from build123d import *

# Parameters (mm, degrees)
BOSS_EXTRUDE1_DEPTH = 2.54


with BuildPart() as part:
    # Sketch1 → Boss-Extrude1 (new body)
    with BuildSketch(Plane.XY):
        with BuildLine():
            Line((-109.2454, -66.7), (-109.2454, 67.7))
            ThreePointArc((-109.2454, 67.7), (-104.516521825, 79.116521825), (-93.1, 83.8454))
            Line((-93.1, 83.8454), (92.1, 83.8454))
            Line((92.1, 83.8454), (93.1, 83.8454))
            ThreePointArc((93.1, 83.8454), (104.516521825, 79.116521825), (109.2454, 67.7))
            Line((109.2454, 67.7), (109.2454, -66.7))
            Line((109.2454, -66.7), (109.2454, -67.7))
            ThreePointArc((109.2454, -67.7), (104.516521825, -79.116521825), (93.1, -83.8454))
            Line((93.1, -83.8454), (-92.1, -83.8454))
            Line((-92.1, -83.8454), (-93.1, -83.8454))
            ThreePointArc((-93.1, -83.8454), (-104.516521825, -79.116521825), (-109.2454, -67.7))
            Line((-109.2454, -67.7), (-109.2454, -66.7))
        make_face()
        with BuildLine():
            Line((-104.6734, -66.7), (-104.6734, 67.7))
            ThreePointArc((-104.6734, 67.7), (-101.283629621, 75.883629621), (-93.1, 79.2734))
            Line((-93.1, 79.2734), (92.1, 79.2734))
            Line((92.1, 79.2734), (93.1, 79.2734))
            ThreePointArc((93.1, 79.2734), (101.283629621, 75.883629621), (104.6734, 67.7))
            Line((104.6734, 67.7), (104.6734, -66.7))
            Line((104.6734, -66.7), (104.6734, -67.7))
            ThreePointArc((104.6734, -67.7), (101.283629621, -75.883629621), (93.1, -79.2734))
            Line((93.1, -79.2734), (-92.1, -79.2734))
            Line((-92.1, -79.2734), (-93.1, -79.2734))
            ThreePointArc((-93.1, -79.2734), (-101.283629621, -75.883629621), (-104.6734, -67.7))
            Line((-104.6734, -67.7), (-104.6734, -66.7))
        make_face(mode=Mode.SUBTRACT)
    extrude(amount=-BOSS_EXTRUDE1_DEPTH)


solid = part.part
Here's how the part is built. I have some questions about the finished solid (model axes, mm). A direction names the side the tool comes from. Round coordinates to 2 decimals unless told otherwise and drop trailing zeros. Order: outer loops, then holes, each group sorted by start corner. A loop starts at its lowest first (then second) coordinate and runs counter-clockwise, first axis right, second up. Notation, with made-up numbers: (55.5, 78.25) -> (61.5, 78.25) arc R30 cw to (61.5, 116.25) -> close; hole circle Ø5 at (67, 1). An arc over 180 degrees is marked (long way). Return JSON: item names as keys, results as strings.
Q1. If we section it at B-B on y = -7.5: List the corners of the cut face in (x, z) for me, plus the area to 3 significant figures.
Filled sheet:
{"outline": "(-109.25, -2.54) -> (-104.67, -2.54) -> (-104.67, 0) -> (-109.25, 0) -> close; (104.67, -2.54) -> (109.25, -2.54) -> (109.25, 0) -> (104.67, 0) -> close", "area": "23.2 mm^2"}
Q2. I need wall thicknesses on line 1 along Y through (x, z) = (17.5, -0.9); line 2 along X through (y, z) = (-22.5, -1.35); line 3 along X through (y, z) = (-75, -1.6). Which ranges of each line are inside material? Lowest first, please. Write a range as from..to.
Filled sheet:
{"line 1": "y = -83.85..-79.27, 79.27..83.85", "line 2": "x = -109.25..-104.67, 104.67..109.25", "line 3": "x = -107.5..-102.08, 102.08..107.5"}
Q3. Which directions (+Z, -Z, +X, -X, +Y, -Y) give clear straight access to the entire face, cutting with the end or side of a thin tool? Please do faces 4 (the cylindrical face through (-101.373, 75.793, -1.252)), 5 (the flat face through (1, 81, -2.54)).
Filled sheet:
{"face 4": "+Z, -Z", "face 5": "-Z, +X, -X, +Y, -Y"}
Q4. If we section it at C-C on z = -0.5: List the corners of the cut face in (x, y) for me.
Filled sheet:
{"outline": "(-109.25, -67.7) arc R16.15 ccw to (-93.1, -83.85) -> (93.1, -83.85) arc R16.15 ccw to (109.25, -67.7) -> (109.25, 67.7) arc R16.15 ccw to (93.1, 83.85) -> (-93.1, 83.85) arc R16.15 ccw to (-109.25, 67.7) -> close; hole (-104.67, -67.7) arc R11.57 ccw to (-93.1, -79.27) -> (93.1, -79.27) arc R11.57 ccw to (104.67, -67.7) -> (104.67, 67.7) arc R11.57 ccw to (93.1, 79.27) -> (-93.1, 79.27) arc R11.57 ccw to (-104.67, 67.7) -> close"}
Q5. If we section it at A-A on x = -15: List the corners of the cut face in (y, z) for me.
Filled sheet:
{"outline": "(-83.85, -2.54) -> (-79.27, -2.54) -> (-79.27, 0) -> (-83.85, 0) -> close; (79.27, -2.54) -> (83.85, -2.54) -> (83.85, 0) -> (79.27, 0) -> close"}
Q6. If we mould it in two halves opening along X, with no side actions, what happens to faces 1 (the cylindrical face through (-104.64, 78.99, -1.25)), 2 (the cylindrical face through (104.64, -78.99, -1.25)), 3 (the cylindrical face through (101.373, -75.793, -1.252))? For each: released by +X, released by -X, zero draft, split by the parting line, or undercut.
Filled sheet:
{"face 1": "released by -X", "face 2": "released by +X", "face 3": "undercut"}
